from build123d import *

# Parameters (mm, degrees)
BASPROSKE_W         = 12
BASPROSKE_H         = 32
TOOTHCUT_DEPTH      = 47.818799643
TEETHCUTS_COUNT     = 30
TEETHCUTS_ANGLE     = 348
BORSKE_R            = 10
BORE_DEPTH          = 50.0000508
BOSS_EXTRUDE1_START = -83
SKETCH1_R           = 10
BOSS_EXTRUDE1_DEPTH = 83
SKETCH3_R           = 13.5
BOSS_EXTRUDE2_DEPTH = 5


with BuildPart() as part:
    # BasProSke → Base-Revolve (revolve)
    with BuildSketch(Plane(origin=(0, 0, 0), x_dir=(1, 0, 0), z_dir=(0, 1, 0)), mode=Mode.PRIVATE) as base_revolve_sk:
        with Locations((6, 16)):
            Rectangle(BASPROSKE_W, BASPROSKE_H)
    revolve(base_revolve_sk.sketch.rotate(Axis((-10, 0, 0), (1, 0, 0)), 180), axis=Axis((-10, 0, 0), (1, 0, 0)))

    # TooCutSke → ToothCut (cut, through all)
    with BuildSketch(Plane(origin=(0, 0, 0), x_dir=(0, 0, -1), z_dir=(1, 0, 0))):
        with BuildLine():
            ThreePointArc((0.918551563, 27.483654488), (0, 27.499), (-0.918551563, 27.483654488))
            ThreePointArc((-0.918551563, 27.483654488), (-1.617208176, 29.787801627), (-2.761784709, 31.906093311))
            ThreePointArc((-2.761784709, 31.906093311), (0, 32.0254), (2.761784709, 31.906093311))
            ThreePointArc((2.761784709, 31.906093311), (1.617208176, 29.787801627), (0.918551563, 27.483654488))
        make_face()
    toothcut = extrude(amount=TOOTHCUT_DEPTH, mode=Mode.SUBTRACT)

    # TeethCuts: ToothCut ×30 about axis
    teethcuts_axis = Axis((-10, 0, 0), (1, 0, 0))
    for i in range(1, TEETHCUTS_COUNT):
        add(toothcut.rotate(teethcuts_axis, i * TEETHCUTS_ANGLE / (TEETHCUTS_COUNT - 1)), mode=Mode.SUBTRACT)

    # BorSke → Bore (cut, symmetric)
    with BuildSketch(Plane(origin=(0, 0, 0), x_dir=(0, 0, -1), z_dir=(1, 0, 0))):
        with Locations(Location((0, 0, 0), (0, 0, 180))):
            Circle(BORSKE_R)
    extrude(amount=BORE_DEPTH, both=True, mode=Mode.SUBTRACT)

    # Sketch1 → Boss-Extrude1 (add)
    with BuildSketch(Plane.ZY.offset(BOSS_EXTRUDE1_START)):
        Circle(SKETCH1_R)
    extrude(amount=BOSS_EXTRUDE1_DEPTH)

    # Sketch3 → Boss-Extrude2 (add)
    with BuildSketch(Plane(origin=(12, 0, 0), x_dir=(0, 0, -1), z_dir=(1, 0, 0))):
        with Locations(Location((0, 0, 0), (0, 0, 180))):
            Circle(SKETCH3_R)
    extrude(amount=BOSS_EXTRUDE2_DEPTH)


solid = part.part
Source: CAD feature listing. Evaluate the final solid. Frame: model axes, mm. A direction names the side the tool comes from. Give positions to 0.01 mm unless a question says otherwise; leave off trailing zeros. Write each loop counter-clockwise with the first axis right and the second up, starting at its lowest first coordinate (ties: lowest second). Pieces come first, ordered by that corner, then holes. Notation, with made-up numbers: (-4.5, 84.5) - (26.5, 84.5) arc R22 ccw to (26.5, 123.5) - close; hole circle Ø11 at (65, 36.25). An arc over 180 degrees is marked (long way). Write item = value, one per line. Start each with the question number.
Q1. Draft query along Y for faces 5 (the cylindrical face through (5.916, -4.699, 29.413)), 6 (the cylindrical face through (5.916, -28.761, -7.748)), 7 (the cylindrical face through (5.916, 29.743, 1.599)). Return one class per face: +Y half, -Y half, draft (parallel to the pull), parting line (faces both ways), or undercut.
Q2. Material intervals for probe 1 along X at (y, z) = (-23, -14); probe 2 along Z at (x, y) = (76, -3.5); probe 3 along Z at (x, y) = (58, -1.5), sorted ascending.
Q3. Reachability of faces 1 (the cylindrical face through (5.92, 28.82, -7.79)), 2 (the cylindrical face through (5.92, 16.26, -24.96)), 3 (the cylindrical face through (5.916, -18.736, 23.237)), 4 (the cylindrical face through (5.92, 4.73, 29.47)) from +Z, -Z, +X, -X, +Y, -Y: full face, straight path, thin tool, end or side. Return the list, or none.
Q4. Pin query (flat end, axial travel): pin 1 Ø4 at (y, z) = (21, 18) entering from +X; pin 2 Ø5 at (y, z) = (12, -19.5) entering from -X; pin 3 Ø5 at (x, z) = (40, 4.5) entering from -Y; pin 4 Ø1.5 at (x, y) = (49.5, 9.5) entering from -Z. Return the tip coordinate at first contact, or that it passes through.
Q5. Cut plane A-A, the plane x = 47. Return loops of the section in (y, z), then the cut area to 3 significant figures.
Computed values:
q1.face_5 = undercut
q1.face_6 = -Y half
q1.face_7 = +Y half
q2.probe_1 = 0 to 12
q2.probe_2 = -9.37 to 9.37
q2.probe_3 = -9.89 to 9.89
q3.face_1 = +X, -X, +Y
q3.face_2 = -Z, +X, -X
q3.face_3 = +X, -X
q3.face_4 = +Z, +X, -X
q4.pin_1 = 12
q4.pin_2 = 0
q4.pin_3 = -9.8
q4.pin_4 = -4.84
q5.outline = circle Ø20 at (0, 0)
q5.area = 314 mm²
